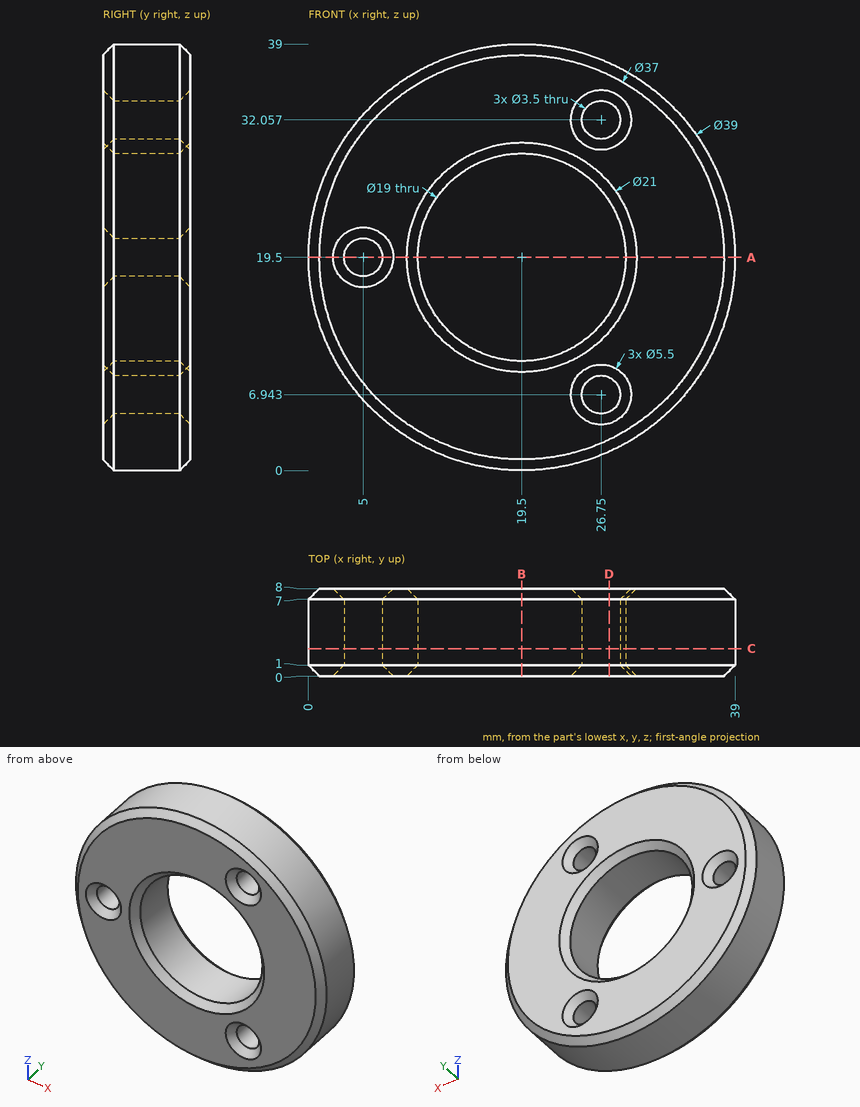
Print and shaded views of the part. All mm, measured from the part's lowest x, y and z. Give positions to 0.01 mm unless a question says otherwise; leave off trailing zeros. Order: outer loops, then holes, each group sorted by start corner. A loop starts at its lowest first (then second) coordinate and runs counter-clockwise, first axis right, second up. Notation, with made-up numbers: M 67,76 L 120,76 A25 cw 120,112 Z; hole C -13.5,69 d11. An arc over 180 degrees is marked long. Use one line per item in the form item = value.
Q1. Slice it at B-B, the plane x = 19.5. Write the cut outline in (y, z), and give its area (3 significant figures).
Conclusion:
outline = M 0,1 L 1,0 L 7,0 L 8,1 L 8,9 L 7,10 L 1,10 L 0,9 Z; M 0,30 L 1,29 L 7,29 L 8,30 L 8,38 L 7,39 L 1,39 L 0,38 Z
area = 156 mm2
Q2. Wall check: probe 1 along Z at (x, y) = (11.5, 1.25) (1 decimal); probe 2 along Z at (x, y) = (24, 6.5) (1 decimal); probe 3 along X at (y, z) = (0.5, 24.5). Give the ranges that are in metal, low to high.
Conclusion:
probe_1 = 1.7 to 14.4, 24.6 to 37.3
probe_2 = 0.5 to 11.1, 27.9 to 38.5
probe_3 = 1.17 to 10.84, 28.16 to 37.83
Q3. Slice it at C-C, the plane y = 2.5. Write the cut outline in (x, z), and give its area (3 significant figures).
Conclusion:
outline = C 19.5,19.5 d39; hole C 5,19.5 d3.5; hole C 19.5,19.5 d19; hole C 26.75,6.94 d3.5; hole C 26.75,32.06 d3.5
area = 882 mm2
Q4. Pin check, flat tips, straight feed: P1, Ø4, axis at x = 12, y = 7, coming from the +Z side; P2, Ø4.5, axis at x = 26.75, z = 6.94, coming from the -Y side; P3, Ø1, axis at x = 9.5, y = 7, coming from the -Z side. Stop position of each tip, or through.
Conclusion:
P1 = 38.21
P2 = 0.5
P3 = 2.47
Q5. Slice it at D-D, the plane x = 27.5. State how many separate pieces and enclosed holes the cut face has, and give its area (3 significant figures).
Conclusion:
separate_pieces = 4
enclosed_holes = 0
area = 142 mm2
Q6. Slice it at A-A, the plane z = 19.5. Write the cut outline in (x, y), and give its area (3 significant figures).
Conclusion:
outline = M 0,1 L 1,0 L 2.25,0 L 3.25,1 L 3.25,7 L 2.25,8 L 1,8 L 0,7 Z; M 6.75,1 L 7.75,0 L 9,0 L 10,1 L 10,7 L 9,8 L 7.75,8 L 6.75,7 Z; M 29,1 L 30,0 L 38,0 L 39,1 L 39,7 L 38,8 L 30,8 L 29,7 Z
area = 126 mm2
